from build123d import *

# Parameters (mm, degrees)
F0_W         = 40
F0_H         = 30
F0_W_2       = 30
F0_H_2       = 24
F4_DEPTH     = 30
F5_SIZE      = 0.2
F6_T1_DEPTH  = 31.0286731952
F6_T3_DEPTH  = 41.0286731952
F6_T5_DEPTH  = 30
F6_T10_DEPTH = 25.0286731952
F6_T16_DEPTH = 25.0286731952
F6_T23_DEPTH = 25.0286731952
F6_T27_DEPTH = 30.225714172
F6_T34_DEPTH = 25.0286731952
F6_T38_DEPTH = 30.225714172
F6_T45_DEPTH = 30.225714172
F6_T49_DEPTH = 25.0286731952
F6_T56_DEPTH = 25.0286731952
F6_T60_DEPTH = 30.225714172


# Not quite as in the source:
# - a fillet or chamfer that OpenCascade refuses, or shapes differently, is made with other operations: its cross-section is extruded or revolved along the edge and cut away or added


with BuildPart() as f2:
    # F2: sweep along a path in F1
    with BuildLine(Plane.XZ) as f2_path:
        Line((0, 0), (0, -4))
    # F0 (on Top) → F2 (sweep)
    with BuildSketch(Plane.XY):
        Rectangle(F0_W, F0_H)
        Rectangle(F0_W_2, F0_H_2, mode=Mode.SUBTRACT)
    sweep(path=f2_path.line)

    # F3 (on face) → F4 (join, through all)
    with BuildSketch(Plane.YZ.offset(-15)):
        Polygon((-10, -2), (-12, 0), (-12, -4), align=None)
        Polygon((10, -2), (12, -4), (12, 0), align=None)
    extrude(amount=F4_DEPTH)

    # F5
    f5_edges = [f2.edges().sort_by_distance(p)[0] for p in [
        (0, -10, -2),
        (0, 10, -2),
    ]]
    chamfer(f5_edges, length=F5_SIZE)

    # F6: chamfer of 0.2 on 8 edges, made by hand

    # F6_s2 → F6_t1 (cut)
    with BuildSketch(Plane.XZ.offset(-15.5143365976)):
        Polygon((19.8, -4), (20, -3.8), (20, -4), align=None)
        Polygon((-19.8, -4), (-20, -3.8), (-20, -4), align=None)
    extrude(amount=F6_T1_DEPTH, mode=Mode.SUBTRACT)

    # F6_s4 → F6_t3 (cut)
    with BuildSketch(Plane.YZ.offset(-20.5143365976)):
        Polygon((-14.8, -4), (-15, -3.8), (-15, -4), align=None)
        Polygon((14.8, -4), (15, -3.8), (15, -4), align=None)
    extrude(amount=F6_T3_DEPTH, mode=Mode.SUBTRACT)

    # F6_s6 → F6_t5 (cut)
    with BuildSketch(Plane.YZ.offset(-15)):
        Polygon((-11.9414213562, -3.9414213562), (-12.0828427125, -4), (-12, -4), align=None)
        Polygon((12.0828427125, -4), (11.9414213562, -3.9414213562), (12, -4), align=None)
    extrude(amount=F6_T5_DEPTH, mode=Mode.SUBTRACT)


with BuildPart() as f6_tool8:
    # F6_s9 → F6_t10 (new body)
    with BuildSketch(Plane.XZ.offset(12.5143365976)):
        Polygon((-15, -3.8), (-15.2, -4), (-15, -4), align=None)
    extrude(amount=-F6_T10_DEPTH)

    split(bisect_by=Plane(origin=(0, -4, 4), x_dir=(1, 0, 0), z_dir=(0, 0.7071067812, -0.7071067812)), keep=Keep.TOP)

    split(bisect_by=Plane(origin=(0, 4, 4), x_dir=(1, 0, 0), z_dir=(0, -0.7071067812, -0.7071067812)), keep=Keep.TOP)


with BuildPart() as f2_1:
    add(f2.part)

    # F6_t7: cut F6_tool8
    add(f6_tool8.part, mode=Mode.SUBTRACT)


with BuildPart() as f6_tool14:
    # F6_s15 → F6_t16 (new body)
    with BuildSketch(Plane.XZ.offset(-12.5143365976)):
        Polygon((15.2, -4), (15, -3.8), (15, -4), align=None)
    extrude(amount=F6_T16_DEPTH)

    split(bisect_by=Plane(origin=(0, -4, 4), x_dir=(1, 0, 0), z_dir=(0, 0.7071067812, -0.7071067812)), keep=Keep.TOP)

    split(bisect_by=Plane(origin=(0, 4, 4), x_dir=(1, 0, 0), z_dir=(0, -0.7071067812, -0.7071067812)), keep=Keep.TOP)


with BuildPart() as f2_2:
    add(f2_1.part)

    # F6_t13: cut F6_tool14
    add(f6_tool14.part, mode=Mode.SUBTRACT)


with BuildPart() as f6_tool21:
    # F6_s22 → F6_t23 (new body)
    with BuildSketch(Plane.XZ.offset(12.5143365976)):
        Polygon((-15, -3.8), (-15.2, -4), (-15, -4), align=None)
    extrude(amount=-F6_T23_DEPTH)

    split(bisect_by=Plane(origin=(0, -4, 4), x_dir=(1, 0, 0), z_dir=(0, -0.7071067812, 0.7071067812)), keep=Keep.TOP)


with BuildPart() as f6_tool25:
    # F6_s26 → F6_t27 (new body)
    with BuildSketch(Plane.YZ.offset(15)):
        Polygon((-11.9414213562, -3.9414213562), (-12.0828427125, -4), (-12, -4), align=None)
    extrude(amount=-F6_T27_DEPTH)

    split(bisect_by=Plane.YZ.offset(-15), keep=Keep.BOTTOM)


with BuildPart() as f6_tool21_1:
    add(f6_tool21.part)

    # F6_t29: intersect F6_tool25
    add(f6_tool25.part, mode=Mode.INTERSECT)


with BuildPart() as f2_3:
    add(f2_2.part)

    # F6_t19: cut F6_tool21
    add(f6_tool21_1.part, mode=Mode.SUBTRACT)


with BuildPart() as f6_tool32:
    # F6_s33 → F6_t34 (new body)
    with BuildSketch(Plane.XZ.offset(12.5143365976)):
        Polygon((-15, -3.8), (-15.2, -4), (-15, -4), align=None)
    extrude(amount=-F6_T34_DEPTH)

    split(bisect_by=Plane(origin=(0, 4, 4), x_dir=(1, 0, 0), z_dir=(0, 0.7071067812, 0.7071067812)), keep=Keep.TOP)


with BuildPart() as f6_tool36:
    # F6_s37 → F6_t38 (new body)
    with BuildSketch(Plane.YZ.offset(-15.225714172)):
        Polygon((12.0828427125, -4), (11.9414213562, -3.9414213562), (12, -4), align=None)
    extrude(amount=F6_T38_DEPTH)

    split(bisect_by=Plane.YZ.offset(-15), keep=Keep.BOTTOM)


with BuildPart() as f6_tool32_1:
    add(f6_tool32.part)

    # F6_t40: intersect F6_tool36
    add(f6_tool36.part, mode=Mode.INTERSECT)


with BuildPart() as f2_4:
    add(f2_3.part)

    # F6_t30: cut F6_tool32
    add(f6_tool32_1.part, mode=Mode.SUBTRACT)


with BuildPart() as f6_tool43:
    # F6_s44 → F6_t45 (new body)
    with BuildSketch(Plane.YZ.offset(15.225714172)):
        Polygon((-11.9414213562, -3.9414213562), (-12.0828427125, -4), (-12, -4), align=None)
    extrude(amount=-F6_T45_DEPTH)

    split(bisect_by=Plane.YZ.offset(15), keep=Keep.TOP)


with BuildPart() as f6_tool47:
    # F6_s48 → F6_t49 (new body)
    with BuildSketch(Plane.XZ.offset(-12.5143365976)):
        Polygon((15.2, -4), (15, -3.8), (15, -4), align=None)
    extrude(amount=F6_T49_DEPTH)

    split(bisect_by=Plane(origin=(0, -4, 4), x_dir=(1, 0, 0), z_dir=(0, -0.7071067812, 0.7071067812)), keep=Keep.TOP)


with BuildPart() as f6_tool43_1:
    add(f6_tool43.part)

    # F6_t51: intersect F6_tool47
    add(f6_tool47.part, mode=Mode.INTERSECT)


with BuildPart() as f2_5:
    add(f2_4.part)

    # F6_t41: cut F6_tool43
    add(f6_tool43_1.part, mode=Mode.SUBTRACT)


with BuildPart() as f6_tool54:
    # F6_s55 → F6_t56 (new body)
    with BuildSketch(Plane.XZ.offset(-12.5143365976)):
        Polygon((15.2, -4), (15, -3.8), (15, -4), align=None)
    extrude(amount=F6_T56_DEPTH)

    split(bisect_by=Plane(origin=(0, 4, 4), x_dir=(1, 0, 0), z_dir=(0, 0.7071067812, 0.7071067812)), keep=Keep.TOP)


with BuildPart() as f6_tool58:
    # F6_s59 → F6_t60 (new body)
    with BuildSketch(Plane.YZ.offset(-15)):
        Polygon((12.0828427125, -4), (11.9414213562, -3.9414213562), (12, -4), align=None)
    extrude(amount=F6_T60_DEPTH)

    split(bisect_by=Plane.YZ.offset(15), keep=Keep.TOP)


with BuildPart() as f6_tool54_1:
    add(f6_tool54.part)

    # F6_t62: intersect F6_tool58
    add(f6_tool58.part, mode=Mode.INTERSECT)


with BuildPart() as f2_6:
    add(f2_5.part)

    # F6_t52: cut F6_tool54
    add(f6_tool54_1.part, mode=Mode.SUBTRACT)


solid = f2_6.part
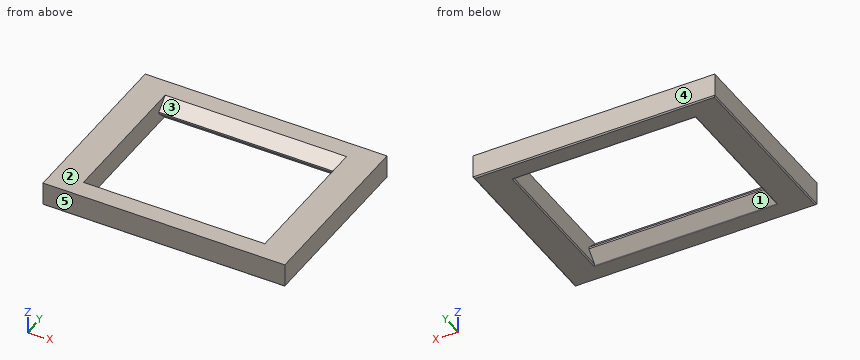
Here's how the part is built. I have some questions about the finished solid (model axes, mm). Face numbers are marked on the shaded views. A direction names the side the tool comes from. Round coordinates to 2 decimals unless told otherwise and drop trailing zeros. Loops run counter-clockwise (first coordinate to the right, second up) from the corner with the lowest first, then second, coordinate; pieces in that order, holes last.
1. If we section it at A-A on x = -8: Write out the boundary of the cut face in (y, z).
Answer list:
outline: (-15, -3.8) - (-14.8, -4) - (-12.08, -4) - (-11.94, -3.94) - (-10.14, -2.14) - (-10.14, -1.86) - (-12, 0) - (-15, 0) - close; (10.14, -2.14) - (11.94, -3.94) - (12.08, -4) - (14.8, -4) - (15, -3.8) - (15, 0) - (12, 0) - (10.14, -1.86) - close
2. Which directions (+Z, -Z, +X, -X, +Y, -Y) give clear straight access to the entire face, cutting with the end or side of a thin tool? Please do the marked faces 1 and 2.
Answer list:
face 1: -Z
face 2: +Z, +X, -X, +Y, -Y
3. If I drill on line 1 along X through (y, z) = (-1, -3.8); line 2 along Y through (x, z) = (10, -2.75); line 3 along Y through (x, z) = (-2, -0.5), over which ranges is the centre line in solid material (lowest first)?
Answer list:
line 1: x = -20 to -15, 15 to 20
line 2: y = -15 to -10.75, 10.75 to 15
line 3: y = -15 to -11.5, 11.5 to 15
4. We'd pull the mould along Y, two halves only. Please class the marked faces 3, 4 and 5: +Y half, -Y half, draft (parallel to the pull), parting line (faces both ways), or undercut.
Answer list:
face 3: undercut
face 4: +Y half
face 5: -Y half
5. If we section it at D-D on z = -2.8: Write out the boundary of the cut face in (x, y), plus the area to 3 significant figures.
Answer list:
outline: (-20, -15) - (20, -15) - (20, 15) - (-20, 15) - close; hole (-15, -10.8) - (15, -10.8) - (15, 10.8) - (-15, 10.8) - close
area: 552 mm2
6. If we section it at B-B on y = 4: Write out the boundary of the cut face in (x, z).
Answer list:
outline: (-20, -3.8) - (-19.8, -4) - (-15.2, -4) - (-15, -3.8) - (-15, 0) - (-20, 0) - close; (15, -3.8) - (15.2, -4) - (19.8, -4) - (20, -3.8) - (20, 0) - (15, 0) - close
7. If we section it at C-C on z = -0.5: Write out the boundary of the cut face in (x, y).
Answer list:
outline: (-20, -15) - (20, -15) - (20, 15) - (-20, 15) - close; hole (-15, -11.5) - (15, -11.5) - (15, 11.5) - (-15, 11.5) - close
